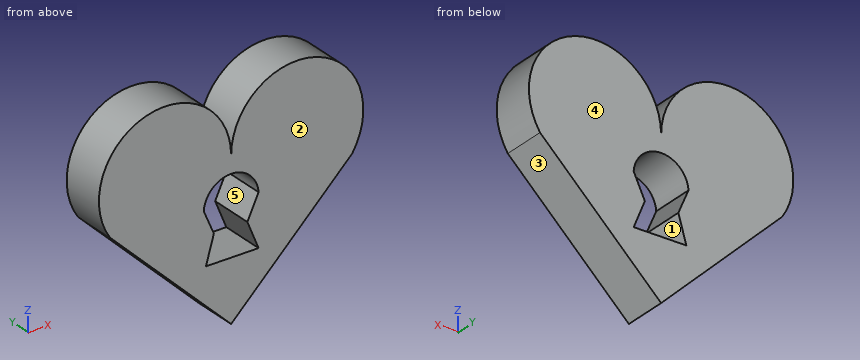
```python
from build123d import *

# Parameters (mm, degrees)
F1_DEPTH = 25.4


with BuildPart() as f1:
    # F0 (on Front) → F1 (new body)
    with BuildSketch(Plane.XZ):
        with BuildLine():
            ThreePointArc((69.798931, 16.962646), (49.142661, 74.564636), (0, 38.1))
            ThreePointArc((0, 38.1), (-49.142661, 74.564636), (-69.798931, 16.962646))
            Line((-69.798931, 16.962646), (0, -50.915454))
            Line((0, -50.915454), (69.798931, 16.962646))
        make_face()
        with BuildLine():
            ThreePointArc((-15.777161, 13.708008), (0.022895, 28.457214), (15.822951, 13.708008))
            Line((15.822951, 13.708008), (9.382167, 0))
            Line((9.382167, 0), (15.822951, -15.835773))
            Line((15.822951, -15.835773), (-14.52887, -15.835773))
            Line((-14.52887, -15.835773), (-9.940196, 0))
            Line((-9.940196, 0), (-15.777161, 13.708008))
        make_face(mode=Mode.SUBTRACT)
    extrude(amount=F1_DEPTH)


solid = f1.part
```
Work out the finished part from the listing and answer in its coordinate system (mm). Face numbers are marked on the shaded views. A direction names the side the tool comes from. Give positions to 0.01 mm unless a question says otherwise; leave off trailing zeros. Order: outer loops, then holes, each group sorted by start corner. A loop starts at its lowest first (then second) coordinate and runs counter-clockwise, first axis right, second up. Notation, with made-up numbers: M 68.5,-30 L 78.5,-30 A16 ccw 78.5,-25 Z; hole C 33,13.5 d5. An arc over 180 degrees is marked long. Return JSON: item names as keys, results as strings.
1) Each of these flat-tipped pins is pushed along its axis until it touches: pin 1 (6 mm diameter, centred on x = 46, y = -4.5, fed in from -Z); pin 2 (8 mm diameter, centred on x = -4, z = 24.5, fed in from -Y); pin 3 (6 mm diameter, centred on x = 47.5, y = -18, fed in from +Z); pin 4 (4 mm diameter, centred on y = -17.5, z = 45, fed in from +X). Where does it stop, or does it pass through?
Resolved:
{"pin 1": "z = -9.1", "pin 2": "y = -25.4", "pin 3": "z = 75.66", "pin 4": "x = 75.88"}
2) Section D-D, the plane x = 18.5 is taken. Write down the section's boundary in (y, z), plus the area to 3 significant figures.
Resolved:
{"outline": "M -25.4,-32.92 L 0,-32.92 L 0,70.77 L -25.4,70.77 Z", "area": "2,630 mm^2"}
3) A tool of negligible diameter and unlimited length cuts with its end or side. For the marked faces 1 and 2, from which of +Z, -Z, +X, -X, +Y, -Y can it reach the whole face along a straight path? Write none if from no direction.
Resolved:
{"face 1": "+Y, -Y", "face 2": "+Z, -Z, +X, -X, -Y"}
4) Section C-C, the plane x = -4 is taken. Write down the section's boundary in (y, z), plus the area to 3 significant figures.
Resolved:
{"outline": "M -25.4,-47.03 L 0,-47.03 L 0,-15.84 L -25.4,-15.84 Z; M -25.4,27.94 L 0,27.94 L 0,55.09 L -25.4,55.09 Z", "area": "1,480 mm^2"}
5) For a pull along X with two mould halves and no side action, classify the marked faces 3, 4 and 5 as +X half, -X half, draft (parallel to the pull), parting line (faces both ways), or undercut.
Resolved:
{"face 3": "+X half", "face 4": "draft", "face 5": "undercut"}
6) Section B-B, the plane z = 3.5 is taken. Write down the section's boundary in (x, y), plus the area to 3 significant figures.
Resolved:
{"outline": "M -55.96,-25.4 L -11.43,-25.4 L -11.43,0 L -55.96,0 Z; M 11.03,-25.4 L 55.96,-25.4 L 55.96,0 L 11.03,0 Z", "area": "2,270 mm^2"}
7) Section A-A, the plane y = -18 is taken. Write down the section's boundary in (x, z), plus the area to 3 significant figures.
Resolved:
{"outline": "M -69.8,16.96 L 0,-50.92 L 69.8,16.96 A38.1 ccw long 0,38.1 A38.1 ccw long Z; hole M -15.78,13.71 L -9.94,0 L -14.53,-15.84 L 15.82,-15.84 L 9.38,0 L 15.82,13.71 A15.84 ccw Z", "area": "11,300 mm^2"}
8) Straight lines are drawn through the part: line 1 along X through (y, z) = (-9, 0.5); line 2 along X through (y, z) = (-8.25, 2); line 3 along Z through (x, y) = (-5, -11). For each, find the intervals that lie inside material, in ascending order. Write a range as [from, to].
Resolved:
{"line 1": "[-52.87, -10.15], [9.62, 52.87]", "line 2": "[-54.41, -10.79], [10.32, 54.41]", "line 3": "[-46.05, -15.84], [27.64, 56.97]"}
